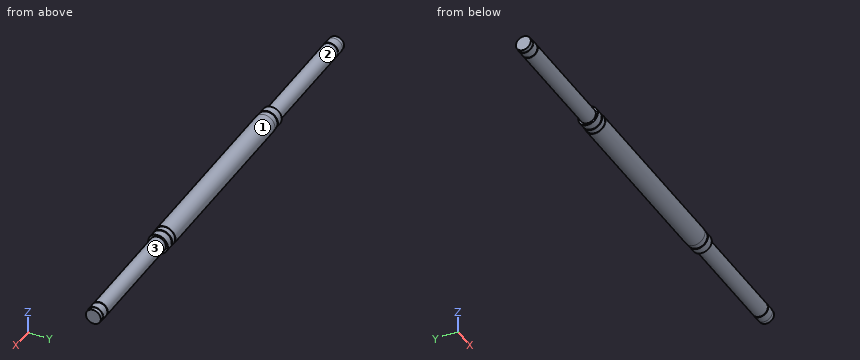
from build123d import *


with BuildPart() as part:
    # 草图1 → 旋转1 (revolve)
    with BuildSketch(Plane(origin=(0, 0, 0), x_dir=(1, 0, 0), z_dir=(0, 1, 0)), mode=Mode.PRIVATE) as revolve_1_sk:
        Polygon((0, 0), (0, 9.5), (5, 9.5), (5, 10), (15, 10), (15, 9.25), (16, 9.25), (16, 10), (156, 10), (156, 12.5), (165.3, 12.5), (165.3, 11.6), (166.5, 11.6), (166.5, 12.5), (173.5, 12.5), (173.5, 13), (413.5, 13), (413.5, 12.5), (420.5, 12.5), (420.5, 11.6), (421.7, 11.6), (421.7, 12.5), (431, 12.5), (431, 10), (571, 10), (571, 9.25), (572, 9.25), (572, 10), (582, 10), (582, 9.5), (587, 9.5), (587, 0), align=None)
    revolve(revolve_1_sk.sketch.rotate(Axis((-75.612934102, 0, 0), (1, 0, 0)), 180), axis=Axis((-75.612934102, 0, 0), (1, 0, 0)))


solid = part.part
Geometry: final body of the model. Coordinates: model frame, mm. Face numbers are marked on the shaded views. A direction names the side the tool comes from. Give positions to 0.01 mm unless a question says otherwise; leave off trailing zeros. Write each loop counter-clockwise with the first axis right and the second up, starting at its lowest first coordinate (ties: lowest second). Pieces come first, ordered by that corner, then holes.
(1) First-contact query: P1, Ø8, axis at x = 316, y = 6.5, coming from the -Z side; P2, Ø1.5, axis at x = 434.5, z = 4, coming from the -Y side; P3, Ø3, axis at x = 507, y = -7, coming from the +Z side. Flat tips, straight axial feed; report the tip coordinate or a pass-through.
(2) Access query for the marked faces 1, 2 and 3. Directions: +Z, -Z, +X, -X, +Y, -Y. A direction counts if a zero-diameter tool reaches every point of the face in a straight line with its end or side. Return the directions, or none.
(3) Ray query, line 1 (X direction, y = 5, z = 8.5); line 2 (X direction, y = 6.25, z = -10); line 3 (X direction, y = 11.25, z = -6.25). Return the intervals inside material, ascending.
(4) Cut plane A-A, the plane x = 217. Return loops of the section in (y, z).
Values follow:
1. P1: stops at z = -12.76
1. P2: stops at y = -9.46
1. P3: stops at z = 8.35
2. face 1: +X, -X
2. face 2: -X
2. face 3: +X
3. line 1: x = 5 to 15, 16 to 571, 572 to 582
3. line 2: x = 156 to 165.3, 166.5 to 420.5, 421.7 to 431
3. line 3: x = 173.5 to 413.5
4. outline: circle Ø26 at (0, 0)
